```python
from build123d import *
from OCP.BRepFilletAPI import BRepFilletAPI_MakeChamfer

# Parameters (mm, degrees)
SKETCH_1_W            = 26
SKETCH_1_H            = 8.5
EXTRUDE_1_DEPTH       = 15
SKETCH_2_W            = 9
SKETCH_2_H            = 17.151512959
CUT_EXTRUDE_2_DEPTH   = 20
CHAMFER_1_SIZE        = 2
CHAMFER_1_SIZE2       = 1.865030172
SKETCH_3_R            = 2
CUT_EXTRUDE_1_DEPTH   = 32.19695498
CHAMFER_2_SIZE        = 2
CHAMFER_2_SIZE2       = 1.865030172
SKETCH_4_W            = 11.3471837
SKETCH_4_H            = 8.882896331
CUT_EXTRUDE_2_2_DEPTH = 4
SKETCH_5_R            = 2
CUT_EXTRUDE_3_DEPTH   = 31.352100422


with BuildPart() as part:
    # Эскиз1 → Вытянуть1 (new body)
    with BuildSketch(Plane.XY):
        with Locations((13, -4.25)):
            Rectangle(SKETCH_1_W, SKETCH_1_H)
    extrude(amount=EXTRUDE_1_DEPTH)

    # Эскиз2 → Cut-Extrude 2 (cut)
    with BuildSketch(Plane(origin=(0, 0, 0), x_dir=(1, 0, 0), z_dir=(0, 1, 0))):
        with Locations((4.5, -12.57575648)):
            Rectangle(SKETCH_2_W, SKETCH_2_H)
        with Locations((21.5, -12.57575648)):
            Rectangle(SKETCH_2_W, SKETCH_2_H)
    extrude(amount=-CUT_EXTRUDE_2_DEPTH, mode=Mode.SUBTRACT)

    # Фаска1
    chamfer_1_edges = [part.edges().sort_by_distance(p)[0] for p in [
        (9, -4.25, 15),
        (17, -4.25, 15),
    ]]
    chamfer_1_side = [part.faces().sort_by_distance(p)[0] for p in [
        (13, -4.25, 15),
    ]]
    chamfer(chamfer_1_edges, length=CHAMFER_1_SIZE, length2=CHAMFER_1_SIZE2, reference=chamfer_1_side[0])

    # Эскиз3 → Вырез-Вытянуть1 (cut, through all)
    with BuildSketch(Plane(origin=(0, 0, 0), x_dir=(-1, 0, 0), z_dir=(0, 0, -1))):
        with Locations((-21, -4.250000001)):
            Circle(SKETCH_3_R)
        with Locations((-5, -4.251501777)):
            Circle(SKETCH_3_R)
    extrude(amount=-CUT_EXTRUDE_1_DEPTH, mode=Mode.SUBTRACT)

    # Фаска2: one chamfer whose edges measure the first distance from different faces: ONE call of the kernel's chamfer builder (chamfer() names one face for all edges)
    chamfer_2_edges_1 = [part.edges().sort_by_distance(p)[0] for p in [
        (23, -4.250000001, 4),
    ]]
    chamfer_2_side_1 = [part.faces().sort_by_distance(p)[0] for p in [
        (23, -4.250000001, 2),
    ]]
    chamfer_2_edges_2 = [part.edges().sort_by_distance(p)[0] for p in [
        (7, -4.251501777, 4),
    ]]
    chamfer_2_side_2 = [part.faces().sort_by_distance(p)[0] for p in [
        (7, -4.251501777, 2),
    ]]
    chamfer_2 = BRepFilletAPI_MakeChamfer(part.part.solid().wrapped)
    for e in chamfer_2_edges_1:
        chamfer_2.Add(CHAMFER_2_SIZE, CHAMFER_2_SIZE2, e.wrapped, chamfer_2_side_1[0].wrapped)  # the first distance lies on this face
    for e in chamfer_2_edges_2:
        chamfer_2.Add(CHAMFER_2_SIZE, CHAMFER_2_SIZE2, e.wrapped, chamfer_2_side_2[0].wrapped)  # the first distance lies on this face
    add(Compound.cast(chamfer_2.Shape()), mode=Mode.REPLACE)

    # Эскиз4 → Cut-Extrude 2 2 (cut)
    with BuildSketch(Plane(origin=(0, 0, 0), x_dir=(1, 0, 0), z_dir=(0, 1, 0))):
        with Locations((13.06322118, -11.410294164)):
            Rectangle(SKETCH_4_W, SKETCH_4_H)
    extrude(amount=-CUT_EXTRUDE_2_2_DEPTH, mode=Mode.SUBTRACT)

    # Эскиз5 → Вырез-Вытянуть3 (cut, through all)
    with BuildSketch(Plane(origin=(0, -4, 0), x_dir=(1, 0, 0), z_dir=(0, 1, 0))):
        with Locations(Location((13, -11.355717768, 0), (0, 0, 270))):
            Circle(SKETCH_5_R)
    extrude(amount=-CUT_EXTRUDE_3_DEPTH, mode=Mode.SUBTRACT)


solid = part.part
```
The model under review builds one solid part; all positions refer to its coordinate system, in mm. A direction names the side the tool comes from. Round coordinates to 2 decimals unless told otherwise and drop trailing zeros. Loops run counter-clockwise (first coordinate to the right, second up) from the corner with the lowest first, then second, coordinate; pieces in that order, holes last.
1) Wall thickness on line 1 along X through (y, z) = (-4.25, 1.4); line 2 along Y through (x, z) = (21, 1.15): over which ranges is each line inside the solid? List them lowest first.
Values follow:
line 1: x = 0 to 3, 7 to 19, 23 to 26
line 2: y = -8.5 to -6.25, -2.25 to 0
2) The part is to be moulded in two halves that separate along X. For faces 1 (the face through (17, -5, 8)), 2 (the face through (13, 0, 3)), 3 (the face through (14.35, -6.22, 9.88)), say which applies: pulls with the +X half, pulls with the -X half, needs draft (parallel to the pull), parting line crosses it, or undercut.
Values follow:
face 1: pulls with the +X half
face 2: needs draft
face 3: undercut
3) Consider section A-A on x = 5. State the section outline as (y, z) points, then the cut area to 3 significant figures.
Values follow:
outline: (-8.5, 0) - (-6.25, 0) - (-6.25, 2) - (-8.12, 4) - (-8.5, 4) - close; (-2.25, 0) - (0, 0) - (0, 4) - (-0.39, 4) - (-2.25, 2) - close
area: 14.3 mm2
4) Clearance check with flat-ended pins moving along their axes: P1, Ø2.5, axis at x = 22, y = -6, coming from the +Z side; P2, Ø2.5, axis at y = -4.5, z = 7, coming from the +X side; P3, Ø4, axis at y = -4.5, z = 9, coming from the -X side. State where each tip first meets the part, or that it passes through.
Values follow:
P1: stops at z = 3.36
P2: stops at x = 17
P3: stops at x = 9
5) Consider section C-C on x = 13. State the section outline as (y, z) points, then the cut area to 3 significant figures.
Values follow:
outline: (-8.5, 0) - (0, 0) - (0, 6.97) - (-4, 6.97) - (-4, 9.36) - (-8.5, 9.36) - close; (-8.5, 13.36) - (-4, 13.36) - (-4, 15) - (-8.5, 15) - close
area: 77.4 mm2
6) Tool access review of faces 4 (the face through (26, -4, 2)), 5 (the face through (1, -2, 4)), 6 (the face through (13, -4, 9)), 7 (the face through (0, -4, 2)), 8 (the face through (25.4, -4.2, 4)): name each direction out of +Z, -Z, +X, -X, +Y, -Y from which nothing blocks a thin tool from reaching the whole face with its end or side.
Values follow:
face 4: +Z, -Z, +X, +Y, -Y
face 5: +Z, -X, +Y, -Y
face 6: +Z, +X, -X, +Y
face 7: +Z, -Z, -X, +Y, -Y
face 8: +Z, +X, +Y, -Y
7) Consider section D-D on y = -4.75. Give the number of separate pieces and of enclosed holes in the cut face, then the cut area to 3 significant figures.
Values follow:
separate pieces: 3
enclosed holes: 1
area: 137 mm2
8) Consider section B-B on z = 10.25. State the section outline as (x, y) points.
Values follow:
outline: (9, -8.5) - (11.33, -8.5) - (11.33, -4) - (9, -4) - close; (14.67, -8.5) - (17, -8.5) - (17, -4) - (14.67, -4) - close
